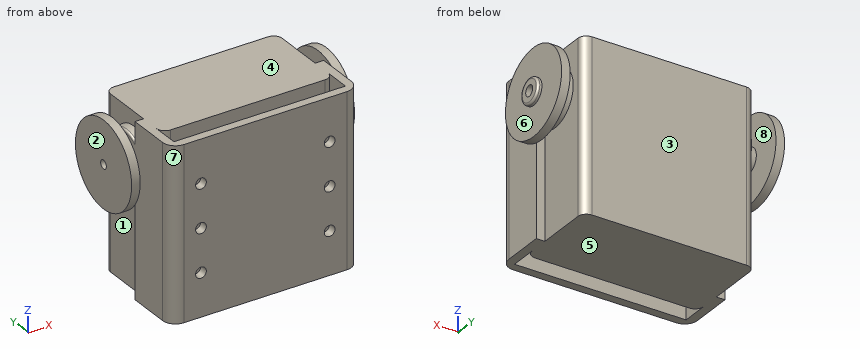
```python
from build123d import *

# Parameters (mm, degrees)
F0_W            = 40
F0_H            = 20.25
F1_DEPTH        = 40
F2_R            = 2
F3_R            = 6.5
F4_DEPTH        = 2
F5_SIZE2        = 0.29999
F5_SIZE         = 1.99999
F6_R            = 0.5
F7_R            = 3
F8_DEPTH        = 4
F9_R            = 0.5
F10_R           = 6.5
F11_DEPTH       = 2
F12_R           = 0.5
F13_R           = 3
F14_DEPTH       = 4
F15_R           = 0.5
F17_D           = 2.5
F17_DEPTH       = 3
F17_CBORE_D     = 2.5
F17_CBORE_DEPTH = 0
F17_TIP         = 0.7510757738
F19_D           = 2.5
F19_DEPTH       = 3
F19_CBORE_D     = 2.5
F19_CBORE_DEPTH = 0
F19_TIP         = 0.7510757738
F21_R           = 10
F21_R_2         = 1
F22_DEPTH       = 2
F24_R           = 10
F24_R_2         = 3
F25_DEPTH       = 2
F27_DEPTH       = 40
F28_R           = 3
F30_D           = 2.5
F30_DEPTH       = 3
F30_TIP         = 0.7510757738


# Not quite as in the source:
# - a fillet or chamfer is up to 0.001 mm smaller than in the source, because OpenCascade refuses the exact size


with BuildPart() as f1:
    # F0 (on Top) → F1 (new body)
    with BuildSketch(Plane.XY):
        Rectangle(F0_W, F0_H)
    extrude(amount=F1_DEPTH)

    # F2
    f2_edges = [f1.edges().sort_by_distance(p)[0] for p in [
        (-20, 10.125, 20),
        (-20, -10.125, 20),
        (20, 10.125, 20),
        (20, -10.125, 20),
    ]]
    fillet(f2_edges, radius=F2_R)

    # F3 (on face) → F4 (join)
    with BuildSketch(Plane(origin=(-20, 0, 0), x_dir=(0, -1, 0), z_dir=(-1, 0, 0))):
        with Locations((0, 30.225)):
            Circle(F3_R)
    extrude(amount=F4_DEPTH)

    # F5 (size 2 and 0.3 in the source; OpenCascade refuses exactly that, so slightly less here)
    f5_edges = [f1.edges().sort_by_distance(p)[0] for p in [
        (-22, 6.5, 30.225),
    ]]
    chamfer(f5_edges, length=F5_SIZE, length2=F5_SIZE2)

    # F6
    f6_edges = [f1.edges().sort_by_distance(p)[0] for p in [
        (-22, 6.20001, 30.225),
    ]]
    fillet(f6_edges, radius=F6_R)

    # F7 (on face) → F8 (join)
    with BuildSketch(Plane(origin=(-22, 0, 0), x_dir=(0, -1, 0), z_dir=(-1, 0, 0))):
        with Locations((0, 30.225)):
            Circle(F7_R)
    extrude(amount=F8_DEPTH)

    # F9
    f9_edges = [f1.edges().sort_by_distance(p)[0] for p in [
        (-26, 3, 30.225),
    ]]
    fillet(f9_edges, radius=F9_R)

    # F10 (on face) → F11 (join)
    with BuildSketch(Plane.YZ.offset(20)):
        with Locations((0, 30.225)):
            Circle(F10_R)
    extrude(amount=F11_DEPTH)

    # F12
    f12_edges = [f1.edges().sort_by_distance(p)[0] for p in [
        (22, -6.5, 30.225),
    ]]
    fillet(f12_edges, radius=F12_R)

    # F13 (on face) → F14 (join)
    with BuildSketch(Plane.YZ.offset(22)):
        with Locations((0, 30.225)):
            Circle(F13_R)
    extrude(amount=F14_DEPTH)

    # F15
    f15_edges = [f1.edges().sort_by_distance(p)[0] for p in [
        (26, -3, 30.225),
    ]]
    fillet(f15_edges, radius=F15_R)

    # F17
    with Locations(Plane(origin=(-26, 0, 0), x_dir=(0, -1, 0), z_dir=(-1, 0, 0))):
        with Locations((0, 30.225)):
            CounterBoreHole(F17_D / 2, F17_CBORE_D / 2, F17_CBORE_DEPTH, depth=F17_DEPTH)
            with Locations((0, 0, -(F17_DEPTH + F17_TIP / 2))):  # 118° drill point
                Cone(0, F17_D / 2, F17_TIP, mode=Mode.SUBTRACT)

    # F19
    with Locations(Plane.YZ.offset(26)):
        with Locations((0, 30.225)):
            CounterBoreHole(F19_D / 2, F19_CBORE_D / 2, F19_CBORE_DEPTH, depth=F19_DEPTH)
            with Locations((0, 0, -(F19_DEPTH + F19_TIP / 2))):  # 118° drill point
                Cone(0, F19_D / 2, F19_TIP, mode=Mode.SUBTRACT)

    # F21 (on offset) → F22 (join)
    with BuildSketch(Plane(origin=(-27, 0, 0), x_dir=(0, -1, 0), z_dir=(-1, 0, 0))):
        with Locations((0, 30.225)):
            Circle(F21_R)
        with Locations((0, 30.225)):
            Circle(F21_R_2, mode=Mode.SUBTRACT)
    extrude(amount=-F22_DEPTH)

    # F24 (on offset) → F25 (join)
    with BuildSketch(Plane.YZ.offset(25)):
        with Locations((0, 30.225)):
            Circle(F24_R)
        with Locations((0, 30.225)):
            Circle(F24_R_2, mode=Mode.SUBTRACT)
    extrude(amount=-F25_DEPTH)

    # F26 (on Top) → F27 (join)
    with BuildSketch(Plane.XY):
        Polygon((22, -16.375), (22, -3.5868030973), (20, -3.5868030973), (20, -14.375), (-20, -14.375), (-20, -3.5868030973), (-22, -3.5868030973), (-22, -16.375), align=None)
    extrude(amount=F27_DEPTH)

    # F28
    f28_edges = [f1.edges().sort_by_distance(p)[0] for p in [
        (22, -16.375, 20),
        (-22, -16.375, 20),
    ]]
    fillet(f28_edges, radius=F28_R)

    # F30
    with Locations(Plane.XZ.offset(16.375)):
        with Locations((-15, 30), (15, 30), (15, 20), (-15, 20), (-15, 10), (15, 10)):
            Hole(F30_D / 2, depth=F30_DEPTH)
            with Locations((0, 0, -(F30_DEPTH + F30_TIP / 2))):  # 118° drill point
                Cone(0, F30_D / 2, F30_TIP, mode=Mode.SUBTRACT)


solid = f1.part
```
Here's how the part is built. I have some questions about the finished solid (model axes, mm). Face numbers are marked on the shaded views. A direction names the side the tool comes from. Round coordinates to 2 decimals unless told otherwise and drop trailing zeros. Write each loop counter-clockwise with the first axis right and the second up, starting at its lowest first coordinate (ties: lowest second). Pieces come first, ordered by that corner, then holes. Notation, with made-up numbers: M -32,5.5 L 11,5.5 A17 ccw 11,35.5 Z; hole C -28,70 d10. An arc over 180 degrees is marked long. Answer as CSV lines item,"result". Start each with the question number.
1. Suppose I cut it at A-A on z = 10. Write out the boundary of the cut face in (x, y) (3 decimals), then the cut area to 3 significant figures.
2. I need wall thicknesses on probe 1 along X at (y, z) = (6.5, 26); probe 2 along Z at (x, y) = (15, -15.4); probe 3 along Y at (x, z) = (12, 6) (3 decimals). Which ranges of each line are inside material? Lowest first, please.
3. Thinking about a two-plate mould opening in X: for the marked faces 1, 2 and 3, which applies, released by +X, released by -X, zero draft, split by the parting line, or undercut?
4. Suppose I cut it at D-D on z = 17.5. Write out the boundary of the cut face in (x, y) (3 decimals).
5. On a 3-axis mill with a long thin cutter (end or side, diameter ignored), from which of +Z, -Z, +X, -X, +Y, -Y can I reach the whole of each face in a straight line? I mean the marked faces 4, 5, 6, 7 and 8. Say none if no direction works.
6. I'm going to push flat-ended pins straight in: pin 1 Ø12 at (y, z) = (-9, 34) entering from +X; pin 2 Ø2 at (y, z) = (-10.5, 25) entering from -X; pin 3 Ø4 at (x, y) = (-3, 3) entering from +Z. Where does each tip first touch, or does it pass through?
7. Suppose I cut it at B-B on x = -15. Write out the boundary of the cut face in (y, z) (3 decimals).
8. Suppose I cut it at C-C on x = 4. Write out the boundary of the cut face in (y, z) (3 decimals).
Check result:
1,outline,"M -22,-13.375 A3 ccw -19,-16.375 L -16.25,-16.375 L -16.25,-14.375 L -20,-14.375 L -20,-8.125 A2 ccw -18,-10.125 L 18,-10.125 A2 ccw 20,-8.125 L 20,-14.375 L 16.25,-14.375 L 16.25,-16.375 L 19,-16.375 A3 ccw 22,-13.375 L 22,-3.587 L 20,-3.587 L 20,8.125 A2 ccw 18,10.125 L -18,10.125 A2 ccw -20,8.125 L -20,-3.587 L -22,-3.587 Z; M -13.75,-16.375 L 13.75,-16.375 L 13.75,-14.375 L -13.75,-14.375 Z"
1,area,"924 mm2"
2,probe 1,"x = -27 to -25, -20 to 20, 23 to 25"
2,probe 2,"z = 0 to 8.75, 11.25 to 18.75, 21.25 to 28.75, 31.25 to 40"
2,probe 3,"y = -16.375 to -14.375, -10.125 to 10.125"
3,face 1,"undercut"
3,face 2,"released by -X"
3,face 3,"zero draft"
4,outline,"M -22,-13.375 A3 ccw -19,-16.375 L 19,-16.375 A3 ccw 22,-13.375 L 22,-3.587 L 20,-3.587 L 20,8.125 A2 ccw 18,10.125 L -18,10.125 A2 ccw -20,8.125 L -20,-3.587 L -22,-3.587 Z; hole M -20,-14.375 L 20,-14.375 L 20,-8.125 A2 cw 18,-10.125 L -18,-10.125 A2 cw -20,-8.125 Z"
5,face 4,"+Z, +Y, -Y"
5,face 5,"-Z, +X, -X, +Y, -Y"
5,face 6,"+X"
5,face 7,"+Z, -Z, -X, -Y"
5,face 8,"none"
6,pin 1,"stops at x = 25"
6,pin 2,"stops at x = -22"
6,pin 3,"stops at z = 40"
7,outline,"M -16.375,0 L -14.375,0 L -14.375,8.75 L -16.375,8.75 Z; M -16.375,11.25 L -14.375,11.25 L -14.375,18.75 L -16.375,18.75 Z; M -16.375,21.25 L -14.375,21.25 L -14.375,28.75 L -16.375,28.75 Z; M -16.375,31.25 L -14.375,31.25 L -14.375,40 L -16.375,40 Z; M -10.125,0 L 10.125,0 L 10.125,40 L -10.125,40 Z"
8,outline,"M -16.375,0 L -14.375,0 L -14.375,40 L -16.375,40 Z; M -10.125,0 L 10.125,0 L 10.125,40 L -10.125,40 Z"
